from build123d import *

# Parameters (mm, degrees)
F0_W     = 127
F0_H     = 9.525
F1_DEPTH = 38.1
F2_DEPTH = 12.7
F3_D     = 22.225
F5_D     = 9.525


with BuildPart() as f1:
    # F0 (on Front) → F1 (new body)
    with BuildSketch(Plane.XZ):
        with Locations((63.5, 4.7625)):
            Rectangle(F0_W, F0_H)
    extrude(amount=F1_DEPTH)

    # F0 (on Front) → F2 (join)
    with BuildSketch(Plane.XZ):
        with BuildLine():
            Line((89.8677585571, 56.4390714728), (0, 9.525))
            Line((0, 9.525), (127, 9.525))
            Line((127, 9.525), (126.9520602505, 34.0146270286))
            ThreePointArc((126.9520602505, 34.0146270286), (114.7182618225, 55.6592523753), (89.8677585571, 56.4390714728))
        make_face()
    extrude(amount=F2_DEPTH)

    # F3 (through all)
    with Locations(Plane(origin=(0, 0, 0), x_dir=(1, 0, 0), z_dir=(0, 1, 0))):
        with Locations((101.6, -33.9649990201)):
            Hole(F3_D / 2)

    # F5 (through all)
    with Locations(Plane.XY.offset(9.525)):
        with Locations((25.4, -25.4), (101.6, -25.4)):
            Hole(F5_D / 2)


solid = f1.part
Model file for the job. Use its own axes, mm. A direction names the side the tool comes from. Round coordinates to 2 decimals unless told otherwise and drop trailing zeros. Loops run counter-clockwise (first coordinate to the right, second up) from the corner with the lowest first, then second, coordinate; pieces in that order, holes last. Notation, with made-up numbers: (-5.5, 27.25) - (16.5, 27.25) arc R34 ccw to (16.5, 62.25) - close; hole circle Ø4 at (82, 63). An arc over 180 degrees is marked (long way). Write each question's results on one line, items separated by ' | '.
(1) Saw through at A-A, the plane x = 101.6. List the corners of the cut face in (y, z) (1 decimal).
Answer below:
outline: (-38.1, 0) - (-30.2, 0) - (-30.2, 9.5) - (-38.1, 9.5) - close; (-20.6, 0) - (0, 0) - (0, 22.9) - (-12.7, 22.9) - (-12.7, 9.5) - (-20.6, 9.5) - close; (-12.7, 45.1) - (0, 45.1) - (0, 59.3) - (-12.7, 59.3) - close
(2) Pin check, flat tips, straight feed: pin 1 (5.5 mm diameter, centred on x = 25.4, y = -25.4, fed in from +Z); pin 2 (25 mm diameter, centred on x = 75.5, z = 38, fed in from -Y); pin 3 (2 mm diameter, centred on y = -10.5, z = 13.5, fed in from +X); pin 4 (1.5 mm diameter, centred on y = -7.5, z = 44, fed in from +X). Stop position of each tip, or through.
Answer below:
pin 1: passes through | pin 2: stops at y = -12.7 | pin 3: stops at x = 126.99 | pin 4: stops at x = 125.19
(3) Mould opens along Y. For faces 1 (the cylindrical face through (97.057, -23.969, 4.696)), 2 (the flat face through (63, -19, 0)), 3 (the flat face through (63, -38.1, 5)) say: released by +Y, released by -Y, zero draft, split by the parting line, or undercut.
Answer below:
face 1: undercut | face 2: zero draft | face 3: released by -Y
(4) 3-axis set-ups, long thin cutter, end or side, ignore diameter. For faces 4 (the cylindrical face through (110.418, -6.439, 40.727)), 5 (the flat face through (77, -12.7, 29)): which of +Z, -Z, +X, -X, +Y, -Y reach the whole face in a straight line?
Answer below:
face 4: +Y, -Y | face 5: +Z, +X, -X, -Y
(5) Wall check: L1, parallel to X at y = -25, z = 7.5; L2, parallel to Y at x = 25.4, z = 3; L3, parallel to Z at x = 101, y = -10. Give the ranges that are in metal, low to high.
Answer below:
L1: x = 0 to 20.65, 30.15 to 96.85, 106.35 to 127 | L2: y = -38.1 to -30.16, -20.64 to 0 | L3: z = 0 to 22.87, 45.06 to 59.31
(6) Saw through at C-C, the plane z = 27.5. List the corners of the cut face in (x, y).
Answer below:
outline: (34.43, -12.7) - (92.56, -12.7) - (92.56, 0) - (34.43, 0) - close; (110.64, -12.7) - (126.96, -12.7) - (126.96, 0) - (110.64, 0) - close
(7) Saw through at D-D, the plane x = 25.4. List the corners of the cut face in (y, z) (1 decimal), then the cut area to 3 significant figures.
Answer below:
outline: (-38.1, 0) - (-30.2, 0) - (-30.2, 9.5) - (-38.1, 9.5) - close; (-20.6, 0) - (0, 0) - (0, 22.8) - (-12.7, 22.8) - (-12.7, 9.5) - (-20.6, 9.5) - close | area: 441 mm^2
(8) Saw through at B-B, the plane y = -25.4. List the corners of the cut face in (x, z) (1 decimal).
Answer below:
outline: (0, 0) - (20.6, 0) - (20.6, 9.5) - (0, 9.5) - close; (30.2, 0) - (96.8, 0) - (96.8, 9.5) - (30.2, 9.5) - close; (106.4, 0) - (127, 0) - (127, 9.5) - (106.4, 9.5) - close
